Geometry: see drawing. Coordinates: mm, zero at the bounding-box minimum. A direction names the side the tool comes from. Coordinates: 2 decimals unless noted, no trailing zeros. Loops run counter-clockwise (first coordinate to the right, second up) from the corner with the lowest first, then second, coordinate; pieces in that order, holes last. Notation, with made-up numbers: (22.5, -1) - (80.5, -1) arc R15 ccw to (80.5, 6) - close; hole circle Ø8 at (21.5, 8). An arc over 180 degrees is marked (long way). Answer in a Markdown table with one row per item.
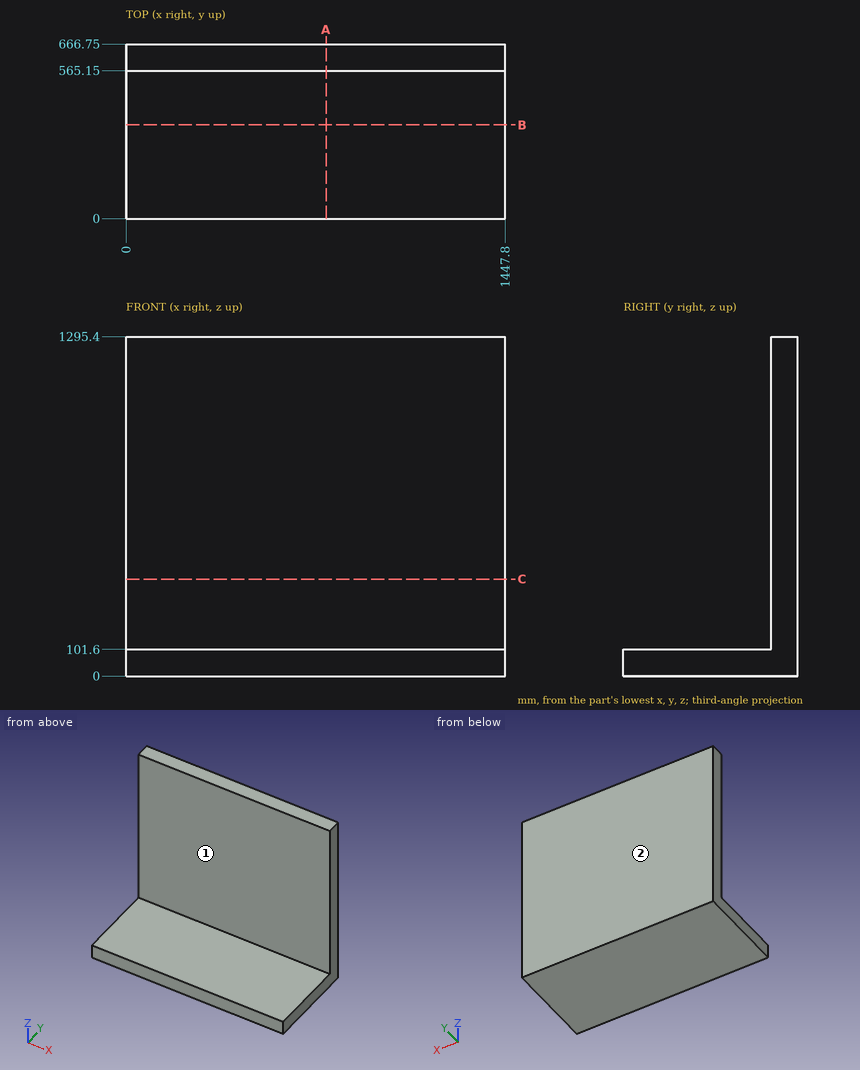
(1) Cut plane C-C on z = 370. Output: boundary loops of the cut face in (x, y).
Verdict:
| item | result |
|---|---|
| outline | (0, 565.15) - (1447.8, 565.15) - (1447.8, 666.75) - (0, 666.75) - close |
(2) Ray query, probe 1 along Y at (x, z) = (707.5, 966.5); probe 2 along Z at (x, y) = (967, 357.5). Return the intervals inside material, ascending.
Verdict:
| item | result |
|---|---|
| probe 1 | y = 565.15 to 666.75 |
| probe 2 | z = 0 to 101.6 |
(3) Cut plane B-B on y = 358. Output: boundary loops of the cut face in (x, z), then the cut area to 3 significant figures.
Verdict:
| item | result |
|---|---|
| outline | (0, 0) - (1447.8, 0) - (1447.8, 101.6) - (0, 101.6) - close |
| area | 147,000 mm² |
(4) Cut plane A-A on x = 764. Output: boundary loops of the cut face in (y, z), then the cut area to 3 significant figures.
Verdict:
| item | result |
|---|---|
| outline | (0, 0) - (666.75, 0) - (666.75, 1295.4) - (565.15, 1295.4) - (565.15, 101.6) - (0, 101.6) - close |
| area | 189,000 mm² |
(5) Access query for the marked faces 1 and 2. Directions: +Z, -Z, +X, -X, +Y, -Y. A direction counts if a zero-diameter tool reaches every point of the face in a straight line with its end or side. Return the directions, or none.
Verdict:
| item | result |
|---|---|
| face 1 | +Z, +X, -X, -Y |
| face 2 | +Z, -Z, +X, -X, +Y |
(6) First-contact query: pin 1 Ø3 at (x, z) = (399, 1124.5) entering from -Y; pin 2 Ø1.5 at (x, y) = (163, 282.5) entering from +Z; pin 3 Ø5 at (x, y) = (810, 564) entering from +Z. Flat tips, straight axial feed; report the tip coordinate or a pass-through.
Verdict:
| item | result |
|---|---|
| pin 1 | stops at y = 565.15 |
| pin 2 | stops at z = 101.6 |
| pin 3 | stops at z = 1295.4 |
